Read the model definition and answer for the solid it produces. Units are mm, in the model's axes. Face numbers are marked on the shaded views. A direction names the side the tool comes from. Coordinates: 2 decimals unless noted, no trailing zeros. Loops run counter-clockwise (first coordinate to the right, second up) from the corner with the lowest first, then second, coordinate; pieces in that order, holes last. Notation, with made-up numbers: (27.25, 65.5) - (84.25, 65.5) arc R20 ccw to (84.25, 81.5) - close; hole circle Ø1 at (17.25, 81). An arc over 180 degrees is marked (long way). Use one line per item in the form item = value.
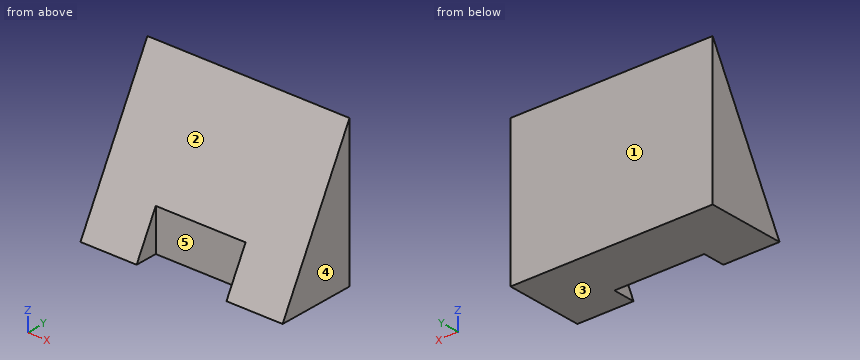
from build123d import *

# Parameters (mm, degrees)
F0_W     = 18
F0_H     = 7
F1_DEPTH = 13
F2_W     = 8
F2_H     = 2
F3_DEPTH = 13.001
F5_DEPTH = 18.001


with BuildPart() as f1:
    # F0 (on Top) → F1 (new body)
    with BuildSketch(Plane.XY):
        with Locations((9, -3.5)):
            Rectangle(F0_W, F0_H)
    extrude(amount=F1_DEPTH)

    # F2 (on face) → F3 (cut, through all)
    with BuildSketch(Plane.XY.offset(13)):
        with Locations((9, -6)):
            Rectangle(F2_W, F2_H)
    extrude(amount=-F3_DEPTH, mode=Mode.SUBTRACT)

    # F4 (on face) → F5 (cut, through all)
    with BuildSketch(Plane.YZ.offset(18)):
        Polygon((-7, 0), (0, 13), (-7, 13), align=None)
    extrude(amount=-F5_DEPTH, mode=Mode.SUBTRACT)


solid = f1.part
Item 1: Which of the six approach directions +Z, -Z, +X, -X, +Y, -Y give full straight-line access (tool end or side, diameter ignored) to the marked faces 4 and 5?
Results below:
face_4 = +Z, -Z, +X, +Y, -Y
face_5 = +Z, -Z, -Y
Item 2: The part is cut by section B-B on z = 3.25. Give the vertices of the cut face in (x, y), plus the area to 3 significant figures.
Results below:
outline = (0, -5.25) - (5, -5.25) - (5, -5) - (13, -5) - (13, -5.25) - (18, -5.25) - (18, 0) - (0, 0) - close
area = 92.5 mm²
Item 3: Find the intervals of material crossed by L1, parallel to Y at x = 13, z = 11.5; L2, parallel to Z at x = 7.5, y = -4; L3, parallel to Z at x = 8.25, y = -3.5, in increasing order.
Results below:
L1 = -0.81 to 0
L2 = 0 to 5.57
L3 = 0 to 6.5
Item 4: For a pull along Y with two mould halves and no side action, classify the marked faces 1, 2 and 3 as +Y half, -Y half, draft (parallel to the pull), parting line (faces both ways), or undercut.
Results below:
face_1 = +Y half
face_2 = -Y half
face_3 = draft
Item 5: The part is cut by section D-D on y = -0.75. Give the vertices of the cut face in (x, z), plus the area to 3 significant figures.
Results below:
outline = (0, 0) - (18, 0) - (18, 11.61) - (0, 11.61) - close
area = 209 mm²
Item 6: The part is cut by section C-C on x = 16.5. Give the vertices of the cut face in (y, z), plus the area to 3 significant figures.
Results below:
outline = (-7, 0) - (0, 0) - (0, 13) - close
area = 45.5 mm²
Item 7: The part is cut by section A-A on y = -5.5. Give the vertices of the cut face in (x, z).
Results below:
outline = (0, 0) - (5, 0) - (5, 2.79) - (0, 2.79) - close; (13, 0) - (18, 0) - (18, 2.79) - (13, 2.79) - close
Item 8: Each of these flat-tipped pins is pushed along its axis until it touches: P1, Ø1.5, axis at x = 9.5, z = 10, coming from the -Y side; P2, Ø2, axis at x = 3.5, z = 2.5, coming from the -Y side; P3, Ø4, axis at x = 7, z = 10.5, coming from the -Y side. Where does it stop, or does it pass through?
Results below:
P1 = -2.02
P2 = -6.19
P3 = -2.42
